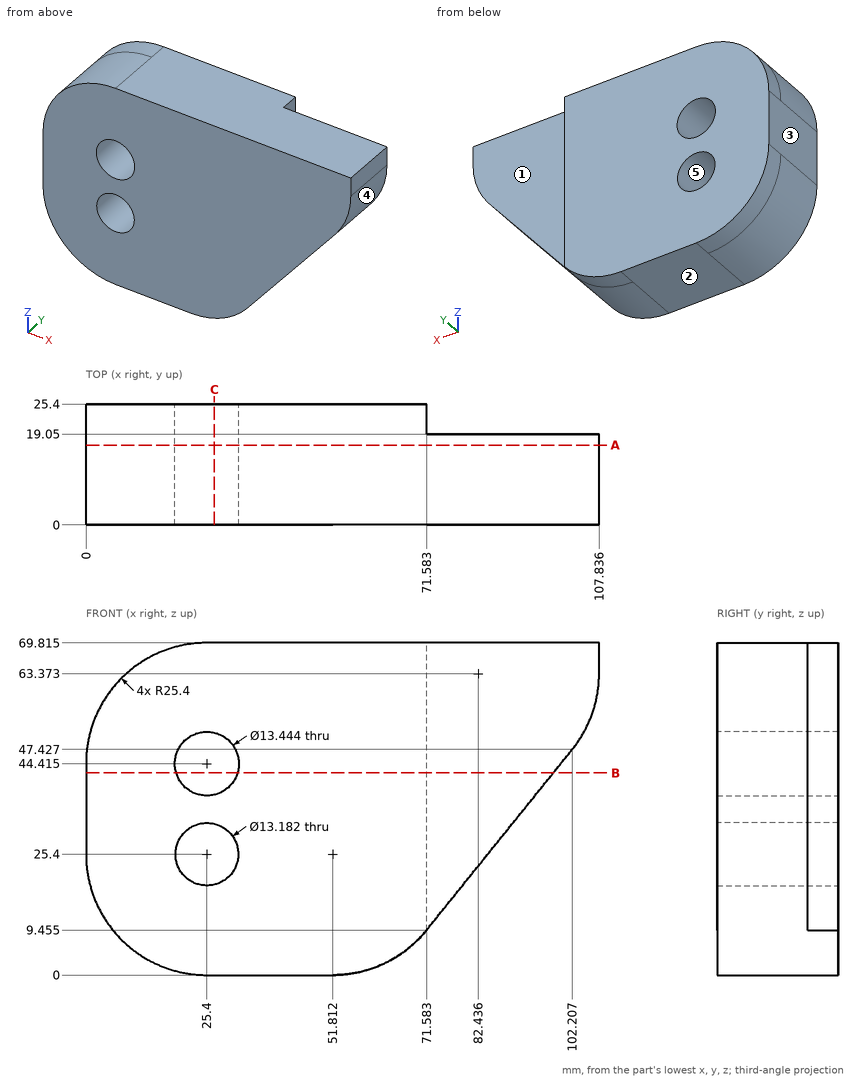
Print and shaded views of the part. All mm, measured from the part's lowest x, y and z. A direction names the side the tool comes from. Give positions to 0.01 mm unless a question says otherwise; leave off trailing zeros. Write each loop counter-clockwise with the first axis right and the second up, starting at its lowest first coordinate (ties: lowest second). Pieces come first, ordered by that corner, then holes. Notation, with made-up numbers: M 58.25,50 L 116.25,50 A24 cw 116.25,69 Z; hole C 83,-34 d7. An arc over 180 degrees is marked long. Use a Markdown table: item, result.
1) Drill centre lines: line 1 (X direction, y = 13.25, z = 26.5); line 2 (Y direction, x = 86.5, z = 39); line 3 (X direction, y = 21.75, z = 20.5) (1 decimal). Where is each one in solid material? Low to high. Write a range as from..to.
Responses:
| item | result |
|---|---|
| line 1 | x = 0..18.9, 31.9..85.33 |
| line 2 | y = 0..19.05 |
| line 3 | x = 0.5..21, 29.8..71.6 |
2) Cut at A-A (y = 16.75). List the corners of the cut face in (x, z) (1 decimal).
Responses:
| item | result |
|---|---|
| outline | M 0,25.4 A25.4 ccw 25.4,0 L 51.8,0 A25.4 ccw 71.6,9.5 L 102.2,47.4 A25.4 ccw 107.8,63.4 L 107.8,69.8 L 25.4,69.8 A25.4 ccw 0,44.4 Z; hole C 25.4,44.4 d13.4; hole C 25.4,25.4 d13.2 |
3) Tool access for the marked faces 1 and 2: list every direction of +Z, -Z, +X, -X, +Y, -Y with a clear straight run to the whole face (end or side of a thin tool).
Responses:
| item | result |
|---|---|
| face 1 | +Z, -Z, +X, +Y |
| face 2 | -Z, +X, -X, +Y, -Y |
4) Pull direction Z, two halves, no side cores. Call the marked faces 3, 4 and 5: +Z half, -Z half, draft (parallel to the pull), parting line (faces both ways), or undercut.
Responses:
| item | result |
|---|---|
| face 3 | draft |
| face 4 | -Z half |
| face 5 | undercut |
5) Cut at C-C (x = 27). List the corners of the cut face in (y, z) (1 decimal), and give its area (3 significant figures).
Responses:
| item | result |
|---|---|
| outline | M 0,0 L 25.4,0 L 25.4,19 L 0,19 Z; M 0,31.8 L 25.4,31.8 L 25.4,37.9 L 0,37.9 Z; M 0,50.9 L 25.4,50.9 L 25.4,69.8 L 0,69.8 Z |
| area | 1,120 mm2 |
6) Pin check, flat tips, straight feed: pin 1 (3 mm diameter, centred on y = 23.5, z = 26, fed in from +X); pin 2 (15.5 mm diameter, centred on x = 25.4, z = 44.42, fed in from -Y); pin 3 (5 mm diameter, centred on x = 74.5, z = 24, fed in from +Y); pin 4 (1 mm diameter, centred on x = 14.5, y = 22, fed in from -Z). Stop position of each tip, or through.
Responses:
| item | result |
|---|---|
| pin 1 | stops at x = 71.58 |
| pin 2 | stops at y = 0 |
| pin 3 | stops at y = 19.05 |
| pin 4 | stops at z = 2.23 |
7) Cut at B-B (z = 42.5). List the corners of the cut face in (x, y), and give its area (3 significant figures).
Responses:
| item | result |
|---|---|
| outline | M 0,0 L 18.96,0 L 18.96,25.4 L 0,25.4 Z; M 31.84,0 L 98.23,0 L 98.23,19.05 L 71.58,19.05 L 71.58,25.4 L 31.84,25.4 Z |
| area | 2,000 mm2 |
